Autodesk Inventor part; units mm, degrees
ref_plane "YZ Plane" through (0, 0, 0) normal (1, 0, 0) x (0, 1, 0)
ref_plane "XZ Plane" through (0, 0, 0) normal (0, 1, 0) x (-1, 0, 0)
ref_plane "XY Plane" through (0, 0, 0) normal (0, 0, 1) x (1, 0, 0)
sketch "Boceto1" plane through (0, 0, 0) normal (0, 1, 0) x (-1, 0, 0)
  line L0 (-1.5, -51.5) -> (1.5, -51.5)
  line L1 (1.5, -51.5) -> (1.5, 51.5)
  line L2 (1.5, 51.5) -> (-1.5, 51.5)
  line L3 (-1.5, 51.5) -> (-1.5, -51.5)
  line L4 (-1.5, -51.5) -> (1.5, 51.5) construction
  line L5 (1.5, -51.5) -> (-1.5, 51.5) construction
  point P0 (0, 0)
  dimension "d0" = 3
  dimension "d1" = 103
extrude "Extrusión1" add sketch "Boceto1" along normal blind 180
sketch "Boceto2" plane through (-1.5, 0, -51.5) normal (-1, 0, 0) x (0, 0, 1)
  line L0 (3, 148.5) -> (100, 148.5)
  line L1 (9.3714, 170) -> (39, 160.0424)
  line L2 (9.3714, 170) -> (93.6286, 170)
  line L3 (51.5, 148.5) -> (51.5, 170)
  circle A0 centre (51.5, 159.25) radius 1.5
  circle A1 centre (93.5, 84) radius 1.5
  circle A2 centre (9.5, 84) radius 1.5
  circle A3 centre (93.5, 6.5) radius 1.25
  circle A4 centre (9.5, 6.5) radius 1.25
  line L4 (3, 0) -> (16, 0)
  line L5 (16, 0) -> (16, 13)
  line L6 (3, 13) -> (16, 13)
  line L7 (3, 0) -> (3, 13)
  circle A5 centre (9.5, 6.5) radius 1.25
  point P0 (51.5, 0)
  dimension "d4" = 3
hole "Agujero1" at (-1.5, 159.25, 0) at (-1.5, 6.5, -42) at (-1.5, 84, -42) at (-1.5, 84, 42) at (-1.5, 6.5, 42) direction (1, 0, 0) diameter 3 depth 5 tip angle 118
sketch "Boceto3" plane through (-1.5, 0, -51.5) normal (-1, 0, 0) x (0, 0, 1)
  circle A0 centre (13.05, 20.58) radius 3.1754
  circle A1 centre (13.05, 47.42) radius 3.1754
  circle A2 centre (42.45, 20.58) radius 3.1754
  circle A3 centre (42.45, 47.42) radius 3.1754
  line L0 (20.6, 69.9) -> (29.6, 69.9)
  line L1 (20.6, 69.9) -> (20.6, 60.9)
  line L2 (20.6, 60.9) -> (29.6, 60.9)
  line L3 (29.6, 60.9) -> (29.6, 69.9)
  circle A4 centre (40.5996, 65.0004) radius 3.4994
  circle A5 centre (62.1002, 64.9998) radius 2.0003
  circle A6 centre (74.6001, 65) radius 2.0001
  circle A7 centre (53, 27) radius 0.75
  circle A8 centre (55.5, 43) radius 1
  circle A9 centre (91.5, 27) radius 1
  circle A10 centre (94.0001, 27) radius 0.7499
  circle A11 centre (93.9999, 43.0001) radius 0.7499
  circle A12 centre (89.575, 56.025) radius 1.0751
  circle A13 centre (89.5749, 71.975) radius 1.0749
  circle A14 centre (13.6251, 71.975) radius 1.0751
  circle A15 centre (13.625, 56.0251) radius 1.0749
  circle A16 centre (53, 43) radius 0.75
  line L4 (30.1, 70.4) -> (20.1, 70.4)
  line L5 (20.1, 70.4) -> (20.1, 60.4)
  line L6 (20.1, 60.4) -> (30.1, 60.4)
  line L7 (30.1, 60.4) -> (30.1, 70.4)
  circle A17 centre (40.5996, 65.0004) radius 4.4994
  circle A18 centre (62.1002, 64.9998) radius 3.0003
  circle A19 centre (74.6001, 65) radius 3.0001
  line L8 (19.6, 59.9) -> (19.6, 70.9)
  line L9 (19.6, 70.9) -> (30.6, 70.9)
  line L10 (30.6, 70.9) -> (30.6, 59.9)
  line L11 (30.6, 59.9) -> (19.6, 59.9)
  line L12 (15.85, 138.4) -> (15.85, 114.4)
  line L13 (87.15, 138.4) -> (15.85, 138.4)
  line L14 (15.85, 114.4) -> (87.15, 114.4)
  line L15 (87.15, 114.4) -> (87.15, 138.4)
  circle A20 centre (14.15, 142.45) radius 1.45
  circle A21 centre (14.15, 111.55) radius 1.45
  circle A22 centre (89.05, 111.55) radius 1.45
  circle A23 centre (89.05, 142.45) radius 1.45
  line L16 (15.35, 138.9) -> (15.35, 113.9)
  line L17 (15.35, 113.9) -> (87.65, 113.9)
  line L18 (87.65, 113.9) -> (87.65, 138.9)
  line L19 (87.65, 138.9) -> (15.35, 138.9)
  circle A24 centre (42.45, 47.42) radius 1.5
  circle A25 centre (13.05, 47.42) radius 1.5
  circle A26 centre (13.05, 20.58) radius 1.5
  circle A27 centre (42.45, 20.58) radius 1.5
  circle A28 centre (14.15, 111.55) radius 1.5
  point P0 (51.5, 0)
  dimension "d12" = 0.5
  dimension "d13" = 1
  dimension "d14" = 1
  dimension "d15" = 1
  dimension "d16" = 0.5
  dimension "d17" = 0.5
  dimension "d18" = 3
  dimension "d19" = 3
  dimension "d20" = 3
  dimension "d21" = 3
  dimension "d22" = 3
extrude "Extrusión2" cut sketch "Boceto3" against normal through all contours L0 L3 L2 L1 | A4 | A5 | A6 | L7 L6 L5 L4 | A17 | A18 | A19 | L8 L9 L10 L11 | L13 L15 L14 L12 | A20 | A21 | A22 | A23 | L19 L18 L17 L16
hole "Agujero2" at (-1.5, 43, -3.5) at (-1.5, 27.0001, -3.5001) at (-1.5, 27, 37.5) at (-1.5, 43, 37.5) direction (1, 0, 0) diameter 2 end through all
sketch "Boceto5" plane through (-1.5, 0, -51.5) normal (-1, 0, 0) x (0, 0, 1)
  circle A0 centre (21.1, 22.5) radius 1.5
  circle A1 centre (21.1, 40.95) radius 1.5
  circle A2 centre (34.5, 40.95) radius 1.5
  circle A3 centre (34.5, 22.5) radius 1.5
  point P0 (51.5, 0)
hole "Agujero3" at (-1.5, 40.95, -17) at (-1.5, 40.95, -30.4) at (-1.5, 22.5, -30.4) at (-1.5, 22.5, -17) direction (1, 0, 0) diameter 3 end through all
properties part number "Panel1"
Build history of the part. All positions in model axes, mm. Coordinates: 2 decimals unless noted, no trailing zeros. Order: outer loops, then holes, each group sorted by start corner. A loop starts at its lowest first (then second) coordinate and runs counter-clockwise, first axis right, second up. Notation, with made-up numbers: (32, 5.25) - (74, 5.25) arc R30 ccw to (74, 28.25) - close; hole circle Ø9 at (46.5, -27.75). An arc over 180 degrees is marked (long way). Write item = value, one per line. Start each with the question number.
1) Saw through at A-A on z = 3.5. Write the cut outline in (x, y), then the cut area to 3 significant figures.
2) Saw through at B-B on y = 131.5. Write the cut outline in (x, z), then the cut area to 3 significant figures.
3) Two-plate mould, pull along Y, no slides. Class faces 1 (the face through (0, 68, 23)), 2 (the face through (-1.5, 89, -1)): pulls with the +Y half, pulls with the -Y half, needs draft (parallel to the pull), parting line crosses it, or undercut.
4) Wall check: line 1 along Y through (x, z) = (0.3, 42); line 2 along Y through (x, z) = (0, -23.5); line 3 along Y through (x, z) = (0.35, -17). Give the ranges that are in metal, low to high. Write a range as from..to.
5) Flat gauge pins, fed straight in: pin 1 Ø8 at (y, z) = (134.5, -23.5) entering from -X; pin 2 Ø8 at (y, z) = (65, 23.1) entering from +X. Where does each tip first touch, or does it go through?
6) Saw through at C-C on z = -8.5. Write the cut outline in (x, y).
7) Saw through at D-D on x = 0.85. Count the separate pieces of the cut face and the enclosed holes in it, then the cut area to 3 significant figures.
From the geometry:
q1.outline = (-1.5, 0) - (1.5, 0) - (1.5, 113.9) - (-1.5, 113.9) - close; (-1.5, 138.9) - (1.5, 138.9) - (1.5, 180) - (-1.5, 180) - close
q1.area = 465 mm^2
q2.outline = (-1.5, -51.5) - (1.5, -51.5) - (1.5, -36.15) - (-1.5, -36.15) - close; (-1.5, 36.15) - (1.5, 36.15) - (1.5, 51.5) - (-1.5, 51.5) - close
q2.area = 92.1 mm^2
q3.face_1 = undercut
q3.face_2 = needs draft
q4.line_1 = 0..5, 8..82.5, 85.5..180
q4.line_2 = 0..59.9, 70.9..113.9, 138.9..180
q4.line_3 = 0..21, 24..39.45, 42.45..113.9, 138.9..180
q5.pin_1 = through
q5.pin_2 = 1.5
q6.outline = (-1.5, 0) - (1.5, 0) - (1.5, 61.19) - (-1.5, 61.19) - close; (-1.5, 68.81) - (1.5, 68.81) - (1.5, 113.9) - (-1.5, 113.9) - close; (-1.5, 138.9) - (1.5, 138.9) - (1.5, 180) - (-1.5, 180) - close
q7.separate_pieces = 1
q7.enclosed_holes = 22
q7.area = 16,400 mm^2
